```python
from build123d import *

# Parameters (mm, degrees)
SKETCH_1_W          = 38
SKETCH_1_H          = 30
EXTRUDE_1_DEPTH     = 20
SKETCH_2_OUTSIDE_W  = 42.476
SKETCH_2_OUTSIDE_H  = 32.476
CUT_EXTRUDE_1_DEPTH = 50.18334813
CUT_EXTRUDE_2_DEPTH = 3.213938048
SKETCH_5_R          = 1
CUT_EXTRUDE_3_DEPTH = 50.18334813
SKETCH_6_R          = 2
CUT_EXTRUDE_4_DEPTH = 41.211951058
SKETCH_7_R          = 1.5
CUT_EXTRUDE_5_DEPTH = 41.211951058
FILLET_1_R          = 2


with BuildPart() as part:
    # 草图1 → 凸台-拉伸1 (new body)
    with BuildSketch(Plane(origin=(0, 0, 0), x_dir=(1, 0, 0), z_dir=(0, 1, 0))):
        with Locations((-8.44083225, -8.979193758)):
            Rectangle(SKETCH_1_W, SKETCH_1_H)
    extrude(amount=EXTRUDE_1_DEPTH)

    # 草图2 outside → 切除-拉伸1 (cut, through all)
    with BuildSketch(Plane.ZY.offset(27.44083225)):
        with Locations((8.979, 10)):
            Rectangle(SKETCH_2_OUTSIDE_W, SKETCH_2_OUTSIDE_H)
        Polygon((23.979193758, 3), (-3.108138222, 3), (17.151672852, 20), (12.151672852, 20), (-6.020806242, 4.751479495), (-6.020806242, 0), (23.979193758, 0), align=None, mode=Mode.SUBTRACT)
    extrude(amount=-CUT_EXTRUDE_1_DEPTH, mode=Mode.SUBTRACT)

    # 草图4 → 切除-拉伸2 (cut)
    with BuildSketch(Plane(origin=(0, 5.752950958, -4.827299027), x_dir=(1, 0, 0), z_dir=(0, 0.7660444431189813, -0.6427876096865356))):
        Polygon((-24.44083225, -25.994695872), (-24.44083225, 0.558013018), (7.55916775, 0.558013018), (7.55916775, -7.441986982), (10.55916775, -7.441986982), (10.55916775, -25.994695872), align=None)
    extrude(amount=-CUT_EXTRUDE_2_DEPTH, mode=Mode.SUBTRACT)

    # 草图5 → 切除-拉伸3 (cut, through all)
    with BuildSketch(Plane.ZY.offset(27.44083225)):
        with Locations((-0.886376682, 6.863996586)):
            Circle(SKETCH_5_R)
        with Locations((10.599170775, 16.511908257)):
            Circle(SKETCH_5_R)
    extrude(amount=-CUT_EXTRUDE_3_DEPTH, mode=Mode.SUBTRACT)

    # 草图6 → 切除-拉伸4 (cut, through all)
    with BuildSketch(Plane(origin=(0, 3, 0), x_dir=(1, 0, 0), z_dir=(0, 1, 0))):
        with Locations(Location((-8.84513683, -16.485782133, 0), (0, 0, 270))):
            Circle(SKETCH_6_R)
    extrude(amount=-CUT_EXTRUDE_4_DEPTH, mode=Mode.SUBTRACT)

    # 草图7 → 切除-拉伸5 (cut, through all)
    with BuildSketch(Plane(origin=(0, 3, 0), x_dir=(1, 0, 0), z_dir=(0, 1, 0))):
        with Locations(Location((-22.069088403, -3.139744133, 0), (0, 0, 270))):
            Circle(SKETCH_7_R)
        with Locations(Location((5.930911597, -3.139744133, 0), (0, 0, 270))):
            Circle(SKETCH_7_R)
    extrude(amount=-CUT_EXTRUDE_5_DEPTH, mode=Mode.SUBTRACT)

    # 圆角1
    fillet_1_edges = [part.edges().sort_by_distance(p)[0] for p in [
        (-27.44083225, 2.375739747, -6.020806242),
        (10.55916775, 2.375739747, -6.020806242),
        (10.55916775, 1.5, 23.979193758),
        (-27.44083225, 1.5, 23.979193758),
    ]]
    fillet(fillet_1_edges, radius=FILLET_1_R)


solid = part.part
```
Read the model definition and answer for the solid it produces. Units are mm, in the model's axes. A direction names the side the tool comes from. Round coordinates to 2 decimals unless told otherwise and drop trailing zeros. Write each loop counter-clockwise with the first axis right and the second up, starting at its lowest first coordinate (ties: lowest second). Pieces come first, ordered by that corner, then holes. Notation, with made-up numbers: M -37.5,66.25 L 16.5,66.25 A19 ccw 16.5,101.25 Z; hole C 40.5,-17.5 d3. An arc over 180 degrees is marked long. One line per item, written item: value.
Q1. For a pull along Y with two mould halves and no side action, classify faces 1 (the flat face through (9.04, 5.5, -0.13)), 2 (the cylindrical face through (-25.962, 5.888, -1.103)), 3 (the flat face through (-14.16, 5.07, -5.64)), 4 (the flat face through (-27.441, 2.5, 6.2)) as +Y half, -Y half, draft (parallel to the pull), parting line (faces both ways), or undercut.
Data:
face 1: undercut
face 2: undercut
face 3: +Y half
face 4: draft
Q2. Which of the six approach directions +Z, -Z, +X, -X, +Y, -Y give full straight-line access (tool end or side, diameter ignored) to faces 5 (the flat face through (-26, 11.4, 6.9)), 6 (the cylindrical face through (9.96, 2.55, -5.45))?
Data:
face 5: +Z, +X, -X
face 6: -Z, +X, +Y, -Y
Q3. Find section B-B on x = -4.5. Write down the section's boundary in (y, z), plus the area to 3 significant figures.
Data:
outline: M 0,-6.02 L 4.75,-6.02 L 5.39,-5.25 L 2.93,-3.19 L 3,-3.11 L 3,23.98 L 0,23.98 Z
area: 94.0 mm2
Q4. Find section C-C on y = 16. Write down the section's boundary in (x, z).
Data:
outline: M -27.44,7.38 L -24.44,7.38 L -24.44,9.74 L -27.44,9.74 Z; M -27.44,11.46 L -24.44,11.46 L -24.44,12.38 L -27.44,12.38 Z
Q5. Flat-ended cylindrical pins translate along their axes: pin 1 Ø1.5 at (x, z) = (-0.5, 20.5) entering from +Y; pin 2 Ø5 at (x, z) = (5.5, 0.5) entering from +Y; pin 3 Ø3 at (y, z) = (6.86, -0.89) entering from -X; pin 4 Ø2.5 at (x, z) = (-22.07, 3.14) entering from -Y. Find the tip coordinate at first contact, or state that the pin passes through.
Data:
pin 1: y = 3
pin 2: y = 10.54
pin 3: x = -27.44
pin 4: through
Q6. Straight lines are drawn through the part: line 1 (Y direction, x = 3, z = 16.25); line 2 (X direction, y = 17, z = 9.5); line 3 (Z direction, x = -23, y = 4). For each, find the intervals that lie inside material, in ascending order. Write a range as [from, to].
Data:
line 1: [0, 3]
line 2: [-27.44, -24.44]
line 3: [-6.02, -4.08]
Q7. Find section A-A on z = 16.25. Write down the section's boundary in (x, y).
Data:
outline: M -27.44,0 L -10.83,0 L -10.83,3 L -27.44,3 Z; M -27.44,19.24 L -24.44,19.24 L -24.44,20 L -27.44,20 Z; M -6.86,0 L 10.56,0 L 10.56,3 L -6.86,3 Z
Q8. Find section D-D on z = 6.5. Write down the section's boundary in (x, y), plus the area to 3 significant figures.
Data:
outline: M -27.44,0 L 10.56,0 L 10.56,3 L -27.44,3 Z; M -27.44,11.06 L -24.44,11.06 L -24.44,15.26 L -27.44,15.26 Z
area: 127 mm2
